from build123d import *

# Parameters (mm, degrees)
F0_W     = 12.8
F0_H     = 6.5
F0_R     = 1
F1_DEPTH = 5.8
F4_W     = 0.9
F4_H     = 3.5
F5_DEPTH = 0.4
F2_W     = 1.2
F2_H     = 2.9
F6_DEPTH = 0.5
F7_R     = 0.4


with BuildPart() as f1:
    # F0 (on Top) → F1 (new body)
    with BuildSketch(Plane.XY):
        with Locations((0.05, 0)):
            Rectangle(F0_W, F0_H)
        with Locations((-3.25, -1.75)):
            Circle(F0_R, mode=Mode.SUBTRACT)
        with Locations((3.25, -1.75)):
            Circle(F0_R, mode=Mode.SUBTRACT)
    extrude(amount=F1_DEPTH)

    # F4 (on offset) → F5 (join)
    with BuildSketch(Plane.XY.offset(2.7)):
        with Locations((-5.08, -5)):
            Rectangle(F4_W, F4_H)
        with Locations((0, -5)):
            Rectangle(F4_W, F4_H)
        with Locations((5.08, -5)):
            Rectangle(F4_W, F4_H)
    extrude(amount=F5_DEPTH)

    # F2 (on face) → F6 (join)
    with BuildSketch(Plane(origin=(0, 3.25, 0), x_dir=(-1, 0, 0), z_dir=(0, 1, 0))):
        with Locations((1.75, 2.95)):
            Rectangle(F2_W, F2_H)
    extrude(amount=F6_DEPTH)

    # F7
    f7_edges = [f1.edges().sort_by_distance(p)[0] for p in [
        (-2.35, 3.75, 2.95),
        (-1.15, 3.75, 2.95),
    ]]
    fillet(f7_edges, radius=F7_R)


solid = f1.part
Verification items for the finished model (mm, model axes). A direction names the side the tool comes from. Coordinates: 2 decimals unless noted, no trailing zeros. Loops run counter-clockwise (first coordinate to the right, second up) from the corner with the lowest first, then second, coordinate; pieces in that order, holes last. Notation, with made-up numbers: (1.5, 24.25) -> (18.5, 24.25) arc R23 cw to (18.5, 40.25) -> close; hole circle Ø10 at (-27.75, -34.5). An arc over 180 degrees is marked (long way). Answer as CSV lines item,"result".
1) Cross-section at C-C, the plane x = -3.25. Record the cut outline in (y, z), then the cut area to 3 significant figures.
Found:
outline,"(-3.25, 0) -> (-2.75, 0) -> (-2.75, 5.8) -> (-3.25, 5.8) -> close; (-0.75, 0) -> (3.25, 0) -> (3.25, 5.8) -> (-0.75, 5.8) -> close"
area,"26.1 mm2"
2) Cross-section at A-A, the plane y = -5.75. Record the cut outline in (x, z).
Found:
outline,"(-5.53, 2.7) -> (-4.63, 2.7) -> (-4.63, 3.1) -> (-5.53, 3.1) -> close; (-0.45, 2.7) -> (0.45, 2.7) -> (0.45, 3.1) -> (-0.45, 3.1) -> close; (4.63, 2.7) -> (5.53, 2.7) -> (5.53, 3.1) -> (4.63, 3.1) -> close"
3) Thickness scan on L1, parallel to Y at x = -3.25, z = 4; L2, parallel to Y at x = 5.5, z = 2.3; L3, parallel to Z at x = -5, y = -3.5. Record the ranges inside material, lowest first. Write a range as from..to.
Found:
L1,"y = -3.25..-2.75, -0.75..3.25"
L2,"y = -3.25..3.25"
L3,"z = 2.7..3.1"
4) Cross-section at D-D, the plane y = -1.75. Record the cut outline in (x, z).
Found:
outline,"(-6.35, 0) -> (-4.25, 0) -> (-4.25, 5.8) -> (-6.35, 5.8) -> close; (-2.25, 0) -> (2.25, 0) -> (2.25, 5.8) -> (-2.25, 5.8) -> close; (4.25, 0) -> (6.45, 0) -> (6.45, 5.8) -> (4.25, 5.8) -> close"
5) Release check for a two-part mould opening along Y. For faces 1 (the flat face through (0, 0, 0)), 2 (the cylindrical face through (2.46, -2.36, 2.86)) record: +Y half, -Y half, draft (parallel to the pull), parting line (faces both ways), or undercut.
Found:
face 1,"draft"
face 2,"undercut"
6) Tool access check on faces 3 (the flat face through (-5, -5, 3.1)), 4 (the flat face through (0, 0, 5.8)), 5 (the flat face through (-5, -5, 2.7)). Record the directions out of +Z, -Z, +X, -X, +Y, -Y that give a thin tool (end or side, any length) a straight path to the whole face; none if there is none.
Found:
face 3,"+Z, +X, -X, -Y"
face 4,"+Z, +X, -X, +Y, -Y"
face 5,"-Z, +X, -X, -Y"
7) Depth check by flat-ended pin: pin 1 (0.7 mm diameter, centred on x = -5, y = -4.5, fed in from +Z); pin 2 (0.5 mm diameter, centred on x = -5.5, y = -5, fed in from -Z); pin 3 (3 mm diameter, centred on x = 2, z = 3.5, fed in from -Y). Enter the tip coordinate at first touch or a pass-through.
Found:
pin 1,"stops at z = 3.1"
pin 2,"stops at z = 2.7"
pin 3,"stops at y = -3.25"
8) Cross-section at B-B, the plane z = 2. Record the cut outline in (x, y), then the cut area to 3 significant figures.
Found:
outline,"(-6.35, -3.25) -> (6.45, -3.25) -> (6.45, 3.25) -> (-1.15, 3.25) -> (-1.15, 3.35) arc R0.4 ccw to (-1.55, 3.75) -> (-1.95, 3.75) arc R0.4 ccw to (-2.35, 3.35) -> (-2.35, 3.25) -> (-6.35, 3.25) -> close; hole circle Ø2 at (-3.25, -1.75); hole circle Ø2 at (3.25, -1.75)"
area,"77.4 mm2"
